Check sheet for the drawn part. Datum: minimum x, y, z corner. Units: mm. A direction names the side the tool comes from. Round coordinates to 2 decimals unless told otherwise and drop trailing zeros. Write each loop counter-clockwise with the first axis right and the second up, starting at its lowest first coordinate (ties: lowest second). Pieces come first, ordered by that corner, then holes. Notation, with made-up numbers: M 25.5,85.25 L 38.5,85.25 A14 cw 38.5,111.25 Z; hole C 26.25,60.25 d4. An arc over 180 degrees is marked long. One line per item, written item: value. Start each with the question number.
Item 1: Section check C-C, the plane x = 9. Record the cut outline in (y, z), then the cut area to 3 significant figures.
Item 2: Draft check along X on the marked faces 1, 2, 3 and 4. Enter one of: +X half, -X half, draft (parallel to the pull), parting line (faces both ways), or undercut.
Item 3: Section check A-A, the plane y = 4.5. Record the cut outline in (x, z).
Item 4: Tool access check on the marked faces 5, 6 and 7. Record the directions out of +Z, -Z, +X, -X, +Y, -Y that give a thin tool (end or side, any length) a straight path to the whole face; none if there is none.
Item 5: Thickness scan on probe 1 along Z at (x, y) = (17.75, 4.5); probe 2 along Z at (x, y) = (3.5, 4). Record the ranges inside material, lowest first. Write a range as from..to.
Item 6: Gauge pin test, flat ends, axial feed: pin 1 (5 mm diameter, centred on x = 15, z = 2, fed in from -Y); pin 2 (3 mm diameter, centred on y = 2.5, z = 3, fed in from -X); pin 3 (3 mm diameter, centred on x = 13.5, z = 8, fed in from +Y). Record the tip position at first contact, or that the pin passes through.
Item 7: Section check B-B, the plane x = 27. Record the cut outline in (y, z), then the cut area to 3 significant figures.
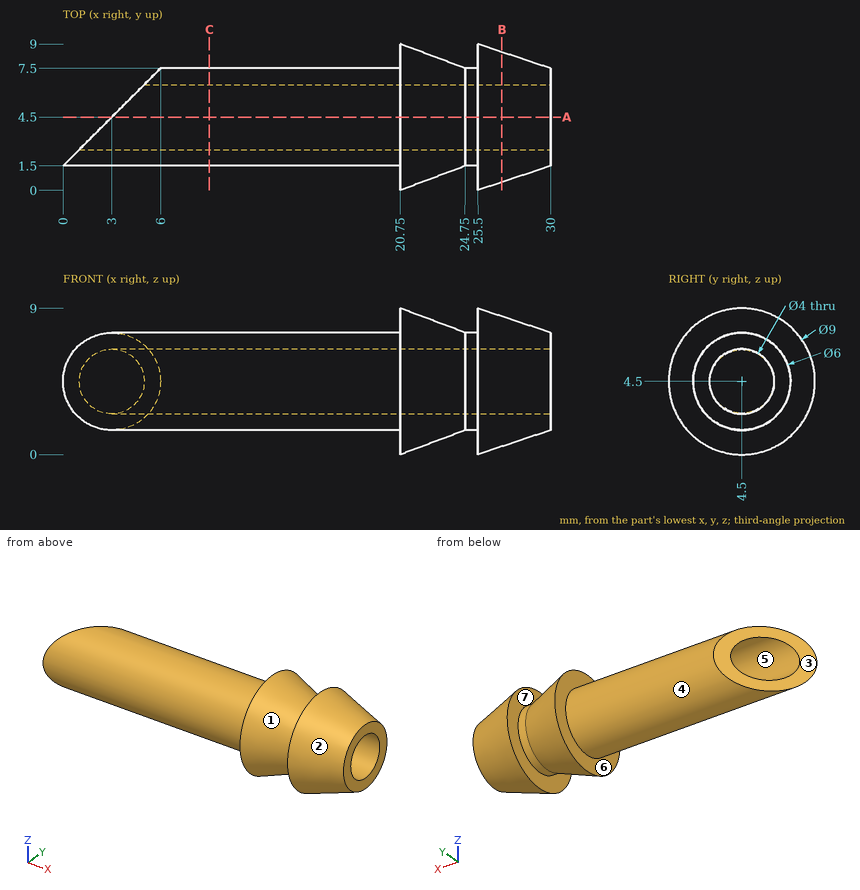
Response values:
1. outline: C 4.5,4.5 d6; hole C 4.5,4.5 d4
1. area: 15.7 mm2
2. face 1: undercut
2. face 2: +X half
2. face 3: -X half
2. face 4: draft
3. outline: M 3,1.5 L 20.75,1.5 L 20.75,0 L 24.75,1.5 L 25.5,1.5 L 25.5,0 L 30,1.5 L 30,2.5 L 3,2.5 Z; M 3,6.5 L 30,6.5 L 30,7.5 L 25.5,9 L 25.5,7.5 L 24.75,7.5 L 20.75,9 L 20.75,7.5 L 3,7.5 Z
4. face 5: +X, -X
4. face 6: -X
4. face 7: none
5. probe 1: z = 1.5..2.5, 6.5..7.5
5. probe 2: z = 1.54..2.56, 6.44..7.46
6. pin 1: stops at y = 1.5
6. pin 2: stops at x = 0.02
6. pin 3: stops at y = 6.74
7. outline: C 4.5,4.5 d8; hole C 4.5,4.5 d4
7. area: 37.7 mm2
